The listing builds one solid part. Answer for the finished solid, in the listing's coordinates (mm). Round coordinates to 2 decimals unless told otherwise and drop trailing zeros. Loops run counter-clockwise (first coordinate to the right, second up) from the corner with the lowest first, then second, coordinate; pieces in that order, holes last. Notation, with made-up numbers: M 3.5,33.25 L 32.5,33.25 A16 ccw 32.5,40.25 Z; hole C -2.5,-9.75 d7. An arc over 180 degrees is marked long. Answer as a JSON object with one key per item and string values.
```python
from build123d import *

# Parameters (mm, degrees)
BOSS_EXTRUDE1_DEPTH = 5
SKETCH2_R           = 1.5
CUT_EXTRUDE1_DEPTH  = 10
SKETCH3_R           = 2
CUT_EXTRUDE2_DEPTH  = 10


with BuildPart() as part:
    # Sketch1 → Boss-Extrude1 (new body)
    with BuildSketch(Plane.XY):
        Polygon((-75, -15), (-70, -15), (-70, -45), (70, -45), (70, -15), (75, -15), (75, 15), (70, 15), (70, 45), (-70, 45), (-70, 15), (-75, 15), align=None)
    extrude(amount=BOSS_EXTRUDE1_DEPTH)

    # Sketch2 → Cut-Extrude1 (cut)
    with BuildSketch(Plane.XY.offset(5)):
        with Locations((15, 18.66)):
            Circle(SKETCH2_R)
        with Locations((15, -9.34)):
            Circle(SKETCH2_R)
        with Locations((-35, 35)):
            Circle(SKETCH2_R)
        with Locations((-35, -14)):
            Circle(SKETCH2_R)
    extrude(amount=-CUT_EXTRUDE1_DEPTH, mode=Mode.SUBTRACT)

    # Sketch3 → Cut-Extrude2 (cut)
    with BuildSketch(Plane.XY.offset(5)):
        with Locations((-72.5, 0)):
            Circle(SKETCH3_R)
        with Locations((72.5, 0)):
            Circle(SKETCH3_R)
    extrude(amount=-CUT_EXTRUDE2_DEPTH, mode=Mode.SUBTRACT)


solid = part.part
```
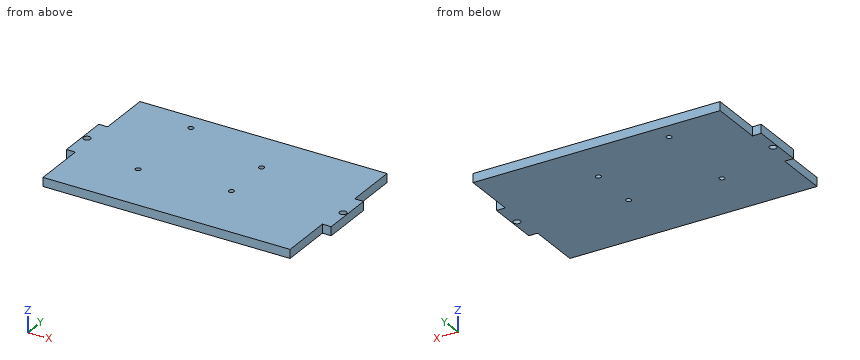
Item 1: Straight lines are drawn through the part: line 1 (Y direction, x = 15, z = 1.95); line 2 (Y direction, x = -72.5, z = 2); line 3 (X direction, y = -8.5, z = 4.85). For each, find the intervals that lie inside material, in ascending order.
Values follow:
{"line 1": "-45 to -10.84, -7.84 to 17.16, 20.16 to 45", "line 2": "-15 to -2, 2 to 15", "line 3": "-75 to 13.76, 16.24 to 75"}
Item 2: The part is cut by section D-D (x = -35). Give the vertices of the cut face in (y, z).
Values follow:
{"outline": "M -45,0 L -15.5,0 L -15.5,5 L -45,5 Z; M -12.5,0 L 33.5,0 L 33.5,5 L -12.5,5 Z; M 36.5,0 L 45,0 L 45,5 L 36.5,5 Z"}
Item 3: The part is cut by section B-B (y = 35). Give the vertices of the cut face in (x, z).
Values follow:
{"outline": "M -70,0 L -36.5,0 L -36.5,5 L -70,5 Z; M -33.5,0 L 70,0 L 70,5 L -33.5,5 Z"}
Item 4: The part is cut by section C-C (x = -72.5). Give the vertices of the cut face in (y, z), then the cut area to 3 significant figures.
Values follow:
{"outline": "M -15,0 L -2,0 L -2,5 L -15,5 Z; M 2,0 L 15,0 L 15,5 L 2,5 Z", "area": "130 mm^2"}
Item 5: The part is cut by section A-A (z = 3.1). Give the vertices of the cut face in (x, y).
Values follow:
{"outline": "M -75,-15 L -70,-15 L -70,-45 L 70,-45 L 70,-15 L 75,-15 L 75,15 L 70,15 L 70,45 L -70,45 L -70,15 L -75,15 Z; hole C -72.5,0 d4; hole C -35,-14 d3; hole C -35,35 d3; hole C 15,-9.34 d3; hole C 15,18.66 d3; hole C 72.5,0 d4"}
Item 6: Flat-ended cylindrical pins translate along their axes: P1, Ø1.5, axis at y = 29.5, z = 2.5, coming from the -X side; P2, Ø2.5, axis at x = 72.5, y = 0, coming from the -Z side. Find the tip coordinate at first contact, or state that the pin passes through.
Values follow:
{"P1": "x = -70", "P2": "through"}
